The figure shows three views and two pictorial views of one solid part (mm, origin at its lowest corner). Answer the questions. A direction names the side the tool comes from. Coordinates: 2 decimals unless noted, no trailing zeros. Loops run counter-clockwise (first coordinate to the right, second up) from the corner with the lowest first, then second, coordinate; pieces in that order, holes last. Notation, with made-up numbers: M -9,67 L 35,67 A18 ccw 35,97 Z; hole C 26.25,0.5 d6. An arc over 180 degrees is marked long. Answer as a JSON object with one key per item and string values. Group by question number.
1. For the marked faces 1, 2, 3 and 4, determine the directions among +Z, -Z, +X, -X, +Y, -Y from which every point of the face is accessible in a straight line to the end or side of a thin tool.
2. Straight lines are drawn through the part: L1, parallel to Y at x = 0.35, z = 18.25 (1 decimal); L2, parallel to Y at x = 1.15, z = 19.75 (1 decimal); L3, parallel to Z at x = 2.2, y = 2 (1 decimal). For each, find the intervals that lie inside material, in ascending order.
3. A cutting plane is placed at A-A on z = 12.5. Give the vertices of the cut face in (x, y).
4. A cutting plane is placed at C-C on x = 2.75. Give the vertices of the cut face in (y, z) (1 decimal), and give its area (3 significant figures).
5. A cutting plane is placed at D-D on y = 21.5. Give the vertices of the cut face in (x, z) (1 decimal).
6. A cutting plane is placed at B-B on z = 21.75. Give the vertices of the cut face in (x, y).
7. Determine the mould class of the marked faces 5, 6 and 7 for opening direction Y: released by +Y, released by -Y, zero draft, split by the parting line, or undercut.
8. Given pin 1 (2 mm diameter, centred on x = 1.5, y = 22.5, fed in from -Z) (1 decimal); pin 2 (2 mm diameter, centred on x = 2, z = 20, fed in from +Y) (1 decimal); pin 3 (1 mm diameter, centred on x = 3, z = 7, fed in from -Y), each flat-ended and moving along its own axis, determine where each tip first touches the part or whether it passes through.
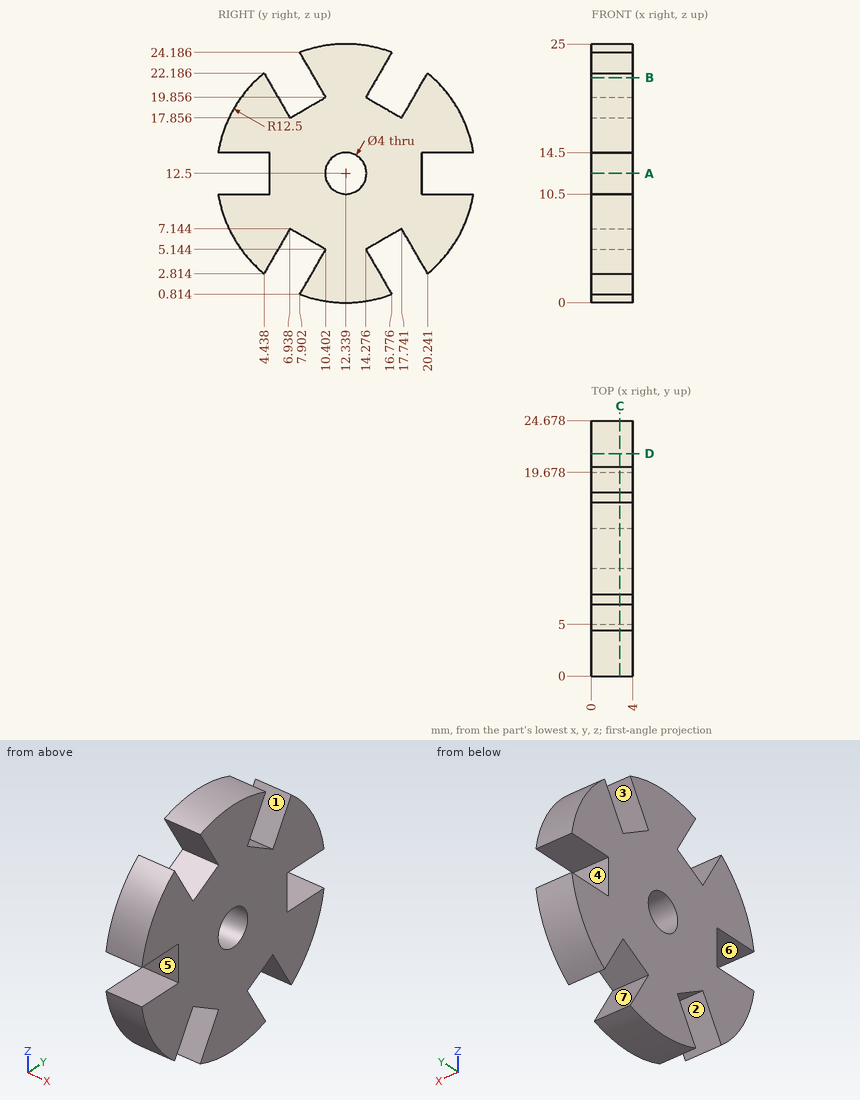
From the geometry:
{
 "1": {"face 1": "+Z, +X, -X", "face 2": "-Z, +X, -X", "face 3": "+X, -X", "face 4": "+X, -X, +Y"},
 "2": {"L1": "y = 1.2 to 6.7, 7.6 to 17.1, 18 to 23.4", "L2": "y = 2.2 to 5.8, 10.2 to 14.5, 18.8 to 22.5", "L3": "z = 5.5 to 10.5, 14.5 to 19.5"},
 "3": {"outline": "M 0,5 L 4,5 L 4,10.34 L 0,10.34 Z; M 0,14.34 L 4,14.34 L 4,19.68 L 0,19.68 Z"},
 "4": {"outline": "M 0,10.5 A12.5 ccw 4.4,2.8 L 6.9,7.1 L 10.4,5.1 L 7.9,0.8 A12.5 ccw 16.8,0.8 L 14.3,5.1 L 17.7,7.1 L 20.2,2.8 A12.5 ccw 24.7,10.5 L 19.7,10.5 L 19.7,14.5 L 24.7,14.5 A12.5 ccw 20.2,22.2 L 17.7,17.9 L 14.3,19.9 L 16.8,24.2 A12.5 ccw 7.9,24.2 L 10.4,19.9 L 6.9,17.9 L 4.4,22.2 A12.5 ccw 0,14.5 L 5,14.5 L 5,10.5 Z; hole C 12.3,12.5 d4", "area": "356 mm²"},
 "5": {"outline": "M 0,4 L 4,4 L 4,10.5 L 0,10.5 Z; M 0,14.5 L 4,14.5 L 4,21 L 0,21 Z"},
 "6": {"outline": "M 0,3.93 L 4,3.93 L 4,4.69 L 0,4.69 Z; M 0,9.31 L 4,9.31 L 4,15.37 L 0,15.37 Z; M 0,19.99 L 4,19.99 L 4,20.75 L 0,20.75 Z"},
 "7": {"face 5": "released by -Y", "face 6": "zero draft", "face 7": "undercut"},
 "8": {"pin 1": "stops at z = 4", "pin 2": "stops at y = 23", "pin 3": "stops at y = 0.88"}
}
